Read the model definition and answer for the solid it produces. Units are mm, in the model's axes. A direction names the side the tool comes from. Coordinates: 2 decimals unless noted, no trailing zeros. Write each loop counter-clockwise with the first axis right and the second up, starting at its lowest first coordinate (ties: lowest second). Pieces come first, ordered by that corner, then holes.
1) The part is cut by section D-D (x = 14.5). Determine the outline of the cut face in (y, z), then the cut area to 3 significant figures.
2) Find the intervals of material crossed by line 1 (Z direction, x = 26, y = 21.5); line 2 (Z direction, x = -5, y = -3); line 3 (Z direction, x = 2.75, y = 31.52), in increasing order.
3) Determine the mould class of faces 1 (the face through (-10, -2, 21)), 2 (the face through (40.82, 22.11, 21.36)), 3 (the face through (41, 0, 21)), 4 (the face through (4.603, 36.477, 20.549)) for opening direction Y: +Y half, -Y half, draft (parallel to the pull), parting line (faces both ways), or undercut.
4) The part is cut by section B-B (x = -5). Determine the outline of the cut face in (y, z).
5) The part is cut by section A-A (z = -5). Determine the outline of the cut face in (x, y).
6) Which of the six approach directions +Z, -Z, +X, -X, +Y, -Y give full straight-line access (tool end or side, diameter ignored) to faces 5 (the face through (52.276, 22, 21)), 6 (the face through (26, 24, 42.4)), 7 (the face through (26, -2, 37.4))?
7) The part is cut by section C-C (y = 24). Determine the outline of the cut face in (x, z), then the cut area to 3 significant figures.
8) Each of these flat-tipped pins is pushed along its axis until it touches: pin 1 Ø23.5 at (x, y) = (35.5, 32.5) entering from -Z; pin 2 Ø10 at (y, z) = (19, 41) entering from -X; pin 3 Ø23.5 at (x, y) = (35.5, 18) entering from +Z. Where does it stop, or does it pass through?
Autodesk Inventor part; units mm, degrees
ref_plane "YZ Plane" through (0, 0, 0) normal (1, 0, 0) x (0, 1, 0)
ref_plane "XZ Plane" through (0, 0, 0) normal (0, 1, 0) x (-1, 0, 0)
ref_plane "XY Plane" through (0, 0, 0) normal (0, 0, 1) x (1, 0, 0)
sketch "Sketch1" plane through (0, 0, 0) normal (0, 0, 1) x (1, 0, 0)
  line L0 (0, 0) -> (0, 46.52)
  line L1 (0, 46.52) -> (52.2762, 42.9195)
  line L2 (52.2762, 42.9195) -> (52.2762, 0)
  line L3 (52.2762, 0) -> (0, 0)
  dimension "d0" = 46.52
  dimension "d1" = 52.4
  dimension "d2" = 86.06
extrude "Extrusion1" add sketch "Sketch1" along normal blind 42.4
sketch "Sketch2" plane through (0, 0, 0) normal (0, -1, 0) x (1, 0, 0)
  line L0 (0, 0) -> (52.2762, 0)
  line L1 (52.2762, 0) -> (52.2762, 42.4)
  line L2 (0, 42.4) -> (52.2762, 42.4)
  line L3 (0, 0) -> (0, 42.4)
  line L4 (47.2762, 37.4) -> (47.2762, 5)
  line L5 (47.2762, 5) -> (5, 5)
  line L6 (5, 5) -> (5, 37.4)
  line L7 (5, 37.4) -> (47.2762, 37.4)
  line L8 (62.2762, 52.4) -> (62.2762, -10)
  line L9 (62.2762, -10) -> (-10, -10)
  line L10 (-10, -10) -> (-10, 52.4)
  line L11 (-10, 52.4) -> (62.2762, 52.4)
  line L12 (57.2762, 47.4) -> (57.2762, -5) construction
  line L13 (57.2762, -5) -> (-5, -5) construction
  line L14 (-5, -5) -> (-5, 47.4) construction
  line L15 (-5, 47.4) -> (57.2762, 47.4) construction
  circle A0 centre (57.2762, 47.4) radius 2.5
  circle A1 centre (-5, 47.4) radius 2.5
  circle A2 centre (-5, -5) radius 2.5
  circle A3 centre (57.2762, -5) radius 2.5
  dimension "d5" = 5
  dimension "d6" = 10
  dimension "d7" = 5
  dimension "d8" = 5
  dimension "d9" = 5
  dimension "d10" = 5
  dimension "d11" = 5
extrude "Extrusion2" add sketch "Sketch2" along normal blind 5 contours L3 L2 L1 L0 | L8 L9 L10 L11
sketch "Sketch3" plane through (0, 46.52, 42.4) normal (0.0687, 0.9976, 0) x (0.9976, -0.0687, 0)
  line L0 (42.4, 32.4) -> (10, 32.4)
  line L1 (10, 32.4) -> (10, 10)
  line L2 (10, 10) -> (42.4, 10)
  line L3 (42.4, 10) -> (42.4, 32.4)
  line L4 (42.4, 32.4) -> (10, 10) construction
  line L5 (10, 32.4) -> (42.4, 10) construction
  line L6 (52.4, 0) -> (0, 0)
  line L7 (0, 42.4) -> (0, 0)
  point P0 (3.1965, 42.4)
  point P1 (26.2, 21.2)
  dimension "d14" = 32.4
  dimension "d15" = 22.4
  dimension "d16" = 21.2
  dimension "d17" = 26.2
extrude "Extrusion3" cut sketch "Sketch3" against normal through all
sketch "Sketch4" plane through (0, 46.52, 0) normal (-1, 0, 0) x (0, 0, 1)
  circle A0 centre (21.2, -15) radius 5
  line L0 (0, 0) -> (42.4, 0)
  line L1 (0, 0) -> (0, -46.52)
  dimension "d20" = 10
  dimension "d21" = 15
  dimension "d22" = 21.2
extrude "Extrusion4" cut sketch "Sketch4" against normal blind 10
properties part number "sort support V3_3DPrint"
Reported:
1. outline: (-5, -10) - (0, -10) - (0, 0) - (45.52, 0) - (45.52, 10) - (0, 10) - (0, 5) - (-5, 5) - close; (-5, 37.4) - (0, 37.4) - (0, 32.4) - (45.52, 32.4) - (45.52, 42.4) - (0, 42.4) - (0, 52.4) - (-5, 52.4) - close
1. area: 1,060 mm2
2. line 1: z = 0 to 10, 32.4 to 42.4
2. line 2: z = -10 to -7.5, -2.5 to 44.9, 49.9 to 52.4
2. line 3: z = 0 to 16.2, 26.2 to 42.4
3. face 1: draft
3. face 2: +Y half
3. face 3: -Y half
3. face 4: undercut
4. outline: (-5, -10) - (0, -10) - (0, -7.5) - (-5, -7.5) - close; (-5, -2.5) - (0, -2.5) - (0, 44.9) - (-5, 44.9) - close; (-5, 49.9) - (0, 49.9) - (0, 52.4) - (-5, 52.4) - close
5. outline: (-10, -5) - (-7.5, -5) - (-7.5, 0) - (-10, 0) - close; (-2.5, -5) - (54.78, -5) - (54.78, 0) - (-2.5, 0) - close; (59.78, -5) - (62.28, -5) - (62.28, 0) - (59.78, 0) - close
6. face 5: +Z, -Z, +X, +Y
6. face 6: +Z, +X, -X, +Y
6. face 7: -Y
7. outline: (0, 0) - (52.28, 0) - (52.28, 42.4) - (0, 42.4) - close; hole (8.47, 10) - (40.95, 10) - (40.95, 32.4) - (8.47, 32.4) - close
7. area: 1,490 mm2
8. pin 1: stops at z = 0
8. pin 2: stops at x = 0
8. pin 3: stops at z = 42.4
